Here's how the part is built. I have some questions about the finished solid (model axes, mm). Face numbers are marked on the shaded views. A direction names the side the tool comes from. Coordinates: 2 decimals unless noted, no trailing zeros. Order: outer loops, then holes, each group sorted by start corner. A loop starts at its lowest first (then second) coordinate and runs counter-clockwise, first axis right, second up. Notation, with made-up numbers: (25, -2.75) -> (72, -2.75) arc R23 ccw to (72, 24.25) -> close; hole circle Ø1 at (42.25, 6.5). An arc over 180 degrees is marked (long way). One line per item, written item: value. Start each with the question number.
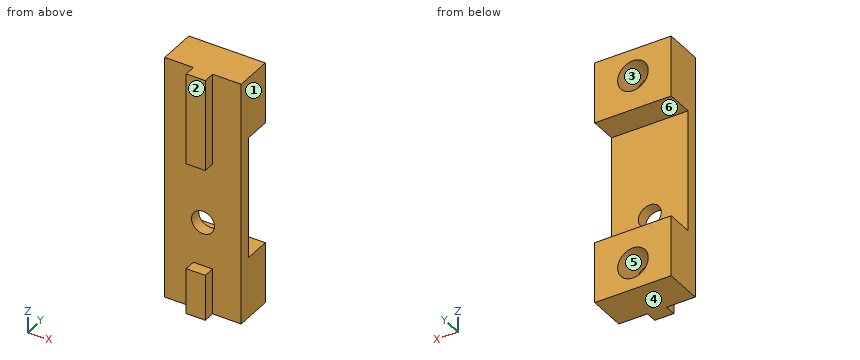
```python
from build123d import *

# Parameters (mm, degrees)
SKETCH1_W               = 20
SKETCH1_H               = 30
BOSS_EXTRUDE1_DEPTH     = 3
SKETCH2_W               = 5
SKETCH2_H               = 12
BOSS_EXTRUDE2_DEPTH     = 3
SKETCH3_R               = 7
SKETCH3_R_2             = 4
BOSS_EXTRUDE3_DEPTH     = 7
SKETCH4_R               = 4
BOSS_EXTRUDE4_DEPTH     = 1
CUT_EXTRUDE1_DEPTH      = 20.339079606
CUT_EXTRUDE1_DEPTH_BACK = 20.339079606
SKETCH5_R               = 3
SKETCH6_R               = 7
SKETCH6_R_2             = 4
BOSS_EXTRUDE6_DEPTH     = 7
SKETCH7_W               = 20
SKETCH7_H               = 3
BOSS_EXTRUDE7_DEPTH     = 19
SKETCH8_W               = 5
SKETCH8_H               = 3
BOSS_EXTRUDE8_DEPTH     = 12
CUT_EXTRUDE2_START      = -1.5
SKETCH10_R              = 4
CUT_EXTRUDE2_DEPTH      = 1.5


with BuildPart() as part:
    # Sketch1 → Boss-Extrude1 (new body)
    with BuildSketch(Plane(origin=(0, 0, 0), x_dir=(1, 0, 0), z_dir=(0, 1, 0))):
        Rectangle(SKETCH1_W, SKETCH1_H)
    boss_extrude1 = extrude(amount=BOSS_EXTRUDE1_DEPTH)

    # Sketch2 → Boss-Extrude2 (add)
    with BuildSketch(Plane.XZ):
        with Locations((0, -9)):
            Rectangle(SKETCH2_W, SKETCH2_H)
    boss_extrude2 = extrude(amount=BOSS_EXTRUDE2_DEPTH)

    # Sketch3 → Boss-Extrude3 (add)
    with BuildSketch(Plane(origin=(0, 3, 0), x_dir=(1, 0, 0), z_dir=(0, 1, 0))):
        with Locations(Location((0, 8, 0), (0, 0, 90))):
            Circle(SKETCH3_R)
        with Locations(Location((0, 8, 0), (0, 0, 270))):
            Circle(SKETCH3_R_2, mode=Mode.SUBTRACT)
    boss_extrude3 = extrude(amount=BOSS_EXTRUDE3_DEPTH)

    # Sketch4 → Boss-Extrude4 (add)
    with BuildSketch(Plane(origin=(0, 3, 0), x_dir=(1, 0, 0), z_dir=(0, 1, 0))):
        with Locations(Location((0, 8, 0), (0, 0, 270))):
            Circle(SKETCH4_R)
    boss_extrude4 = extrude(amount=BOSS_EXTRUDE4_DEPTH)

    # Sketch5 → Cut-Extrude1 (cut, two sides: drawn at the far end of the back side and taken through both)
    with BuildSketch(Plane(origin=(0, 3, 0), x_dir=(1, 0, 0), z_dir=(0, 1, 0)).offset(-CUT_EXTRUDE1_DEPTH_BACK)):
        with Locations(Location((0, -8.5, 0), (0, 0, 90))):
            Circle(SKETCH5_R)
    extrude(amount=CUT_EXTRUDE1_DEPTH + CUT_EXTRUDE1_DEPTH_BACK, mode=Mode.SUBTRACT)

    # Sketch6 → Boss-Extrude6 (add)
    # profile 1 of 2: a face of its own
    with BuildSketch(Plane(origin=(0, 3, 0), x_dir=(1, 0, 0), z_dir=(0, 1, 0))):
        Polygon((0, 15), (-10, 15), (-10, -1), (10, -1), (10, 15), align=None)
        with BuildLine():
            ThreePointArc((7, 8), (-4.949747468, 3.050252532), (0, 15))
            ThreePointArc((0, 15), (4.949747468, 12.949747468), (7, 8))
        make_face(mode=Mode.SUBTRACT)
    # profile 2 of 2: a face of its own
    with BuildSketch(Plane(origin=(0, 3, 0), x_dir=(1, 0, 0), z_dir=(0, 1, 0))):
        with Locations((0, 8)):
            Circle(SKETCH6_R)
        with Locations(Location((0, 8, 0), (0, 0, 270))):
            Circle(SKETCH6_R_2, mode=Mode.SUBTRACT)
    boss_extrude6 = extrude(amount=BOSS_EXTRUDE6_DEPTH)

    # Sketch7 → Boss-Extrude7 (add)
    with BuildSketch(Plane.XY.offset(15)):
        with Locations((0, 1.5)):
            Rectangle(SKETCH7_W, SKETCH7_H)
    extrude(amount=BOSS_EXTRUDE7_DEPTH)

    # Mirror3: Boss-Extrude1, Boss-Extrude2, Boss-Extrude3, Boss-Extrude4, Boss-Extrude6 across plane
    add(boss_extrude1.mirror(Plane.XY.offset(17)))
    add(boss_extrude2.mirror(Plane.XY.offset(17)))
    add(boss_extrude3.mirror(Plane.XY.offset(17)))
    add(boss_extrude4.mirror(Plane.XY.offset(17)))
    add(boss_extrude6.mirror(Plane.XY.offset(17)))

    # Sketch8 → Boss-Extrude8 (add)
    with BuildSketch(Plane(origin=(0, 0, 37), x_dir=(-1, 0, 0), z_dir=(0, 0, -1))):
        with Locations((0, -1.5)):
            Rectangle(SKETCH8_W, SKETCH8_H)
    extrude(amount=BOSS_EXTRUDE8_DEPTH)

    # Sketch10 → Cut-Extrude2 (cut)
    with BuildSketch(Plane(origin=(0, 4, 0), x_dir=(1, 0, 0), z_dir=(0, 1, 0)).offset(CUT_EXTRUDE2_START)):
        with Locations(Location((0, 8, 0), (0, 0, 270))):
            Circle(SKETCH10_R)
        with Locations(Location((0, -42, 0), (0, 0, 90))):
            Circle(SKETCH10_R)
    extrude(amount=CUT_EXTRUDE2_DEPTH, mode=Mode.SUBTRACT)


solid = part.part
```
Q1. I need wall thicknesses on line 1 (X direction, y = 7.75, z = 42); line 2 (Z direction, x = -5, y = 6.25); line 3 (Y direction, x = 2.25, z = 32). Which ranges of each line are inside material? Lowest first, please.
Q2. If we mould it in two halves opening along X, with no side actions, what happens to the marked faces 1, 2 and 3? For each: +X half, -X half, draft (parallel to the pull), parting line (faces both ways), or undercut.
Q3. For the marked faces 4, 5 and 6, which set-ups out of +Z, -Z, +X, -X, +Y, -Y let a thin tool reach every point of the face, with its end or its side?
Q4. Imagine slicing it at A-A (y = 8.75). Write out the boundary of the cut face in (x, z), plus the area to 3 significant figures.
Q5. For P1, Ø7, axis at x = 0, z = 8.5, coming from the +Y side; P2, Ø2.5, axis at y = -1.5, z = 35.5, coming from the -X side; P3, Ø1, axis at x = -3, z = 0.5, coming from the -Y side, each with a flat end and sliding along its axis, tell me the tip position at first contact or that it passes through.
Q6. Imagine slicing it at D-D (y = -2). Write out the boundary of the cut face in (x, z).
Q7. Imagine slicing it at C-C (x = 0). Write out the boundary of the cut face in (y, z), plus the area to 3 significant figures.
Q8. Imagine slicing it at B-B (z = 8.5). Write out the boundary of the cut face in (x, y), plus the area to 3 significant figures.
Completed:
1. line 1: x = -10 to -4, 4 to 10
1. line 2: z = -15 to 1, 33 to 49
1. line 3: y = -3 to 3
2. face 1: +X half
2. face 2: draft
2. face 3: undercut
3. face 4: -Z, +X, -X, +Y, -Y
3. face 5: +Y
3. face 6: +X, -X, +Y
4. outline: (-10, -15) -> (10, -15) -> (10, 1) -> (-10, 1) -> close; (-10, 33) -> (10, 33) -> (10, 49) -> (-10, 49) -> close; hole circle Ø8 at (0, -8); hole circle Ø8 at (0, 42)
4. area: 539 mm2
5. P1: stops at y = 3
5. P2: stops at x = -2.5
5. P3: stops at y = 0
6. outline: (-2.5, -15) -> (2.5, -15) -> (2.5, -3) -> (-2.5, -3) -> close; (-2.5, 25) -> (2.5, 25) -> (2.5, 49) -> (-2.5, 49) -> close
7. outline: (-3, -15) -> (10, -15) -> (10, -12) -> (2.5, -12) -> (2.5, -4) -> (10, -4) -> (10, 1) -> (3, 1) -> (3, 5.5) -> (0, 5.5) -> (0, -3) -> (-3, -3) -> close; (-3, 25) -> (0, 25) -> (0, 11.5) -> (3, 11.5) -> (3, 33) -> (10, 33) -> (10, 38) -> (2.5, 38) -> (2.5, 46) -> (10, 46) -> (10, 49) -> (-3, 49) -> close
7. area: 386 mm2
8. outline: (-10, 0) -> (-3, 0) -> (-3, 3) -> (-10, 3) -> close; (3, 0) -> (10, 0) -> (10, 3) -> (3, 3) -> close
8. area: 42.0 mm2
